For this review, take the finished solid that the model builds, in its own axes (mm). Give positions to 0.01 mm unless a question says otherwise; leave off trailing zeros. Order: outer loops, then holes, each group sorted by start corner. A loop starts at its lowest first (then second) coordinate and runs counter-clockwise, first axis right, second up.
Item 1: The part is to be moulded in two halves that separate along X. For faces 1 (the cylindrical face through (24.369, -22.003, 1.479)), 2 (the cylindrical face through (-29.85, -23.93, 1.52)), 3 (the flat face through (1, -26, 1)), say which applies: released by +X, released by -X, zero draft, split by the parting line, or undercut.
Item 2: For P1, Ø3.5, axis at x = -25, y = -20, coming from the -Z side; P2, Ø5.5, axis at x = -25, y = 20, coming from the -Z side, all flat-tipped, find the tip position at first contact; note any pin that passes through.
Item 3: Consider section D-D (x = 25). Give the boundary of the cut face in (y, z).
Item 4: Consider section B-B (y = 0). Give the boundary of the cut face in (x, z), plus the area to 3 significant figures.
Item 5: Consider section C-C (z = 2). Give the number of separate pieces and of enclosed holes in the cut face, plus the area to 3 significant figures.
Item 6: For probe 1 along Y at (x, z) = (-10, 1); probe 2 along Y at (x, z) = (25, 2.3); probe 3 along X at (y, z) = (0, 1.25), list the stretches that pass through material, from the lowest coordinate up.
Item 7: Consider section A-A (x = 10). Give the boundary of the cut face in (y, z).
Autodesk Inventor part; units mm, degrees
ref_plane "YZ Plane" through (0, 0, 0) normal (1, 0, 0) x (0, 1, 0)
ref_plane "XZ Plane" through (0, 0, 0) normal (0, 1, 0) x (-1, 0, 0)
ref_plane "XY Plane" through (0, 0, 0) normal (0, 0, 1) x (1, 0, 0)
sketch "スケッチ1" plane through (0, 0, 0) normal (0, 0, 1) x (1, 0, 0)
  line L0 (30, -26) -> (-30, -26)
  line L1 (-30, -26) -> (-30, 26)
  line L2 (-30, 26) -> (30, 26)
  line L3 (30, 26) -> (30, -26)
  line L4 (30, -26) -> (-30, 26) construction
  line L5 (-30, -26) -> (30, 26) construction
  point P0 (0, 0)
  dimension "d0" = 60
  dimension "d1" = 52
extrude "押し出し1" add sketch "スケッチ1" along normal blind 3
sketch "スケッチ2" plane through (0, 0, 3) normal (0, 0, 1) x (1, 0, 0)
  line L0 (-10, -20) -> (10, -20)
  line L1 (10, -20) -> (10, 20)
  line L2 (10, 20) -> (-10, 20)
  line L3 (-10, 20) -> (-10, -20)
  line L4 (-10, -20) -> (10, 20) construction
  line L5 (10, -20) -> (-10, 20) construction
  line L6 (-30, -26) -> (30, -26)
  point P0 (0, 0)
  point P1 (0, 20)
  point P2 (0, -20)
  dimension "d4" = 20
  dimension "d5" = 40
  dimension "d6" = 6
hole "穴1" at (-10, 20, 3) at (-10, -20, 3) at (10, -20, 3) at (10, 20, 3) at (0, -20, 3) at (0, 0, 3) at (0, 20, 3) direction (0, 0, -1) diameter 3.3 depth 8.8
sketch "スケッチ4" plane through (0, 0, 3) normal (0, 0, 1) x (1, 0, 0)
  line L0 (-25, -20) -> (25, -20)
  line L1 (25, -20) -> (25, 20)
  line L2 (25, 20) -> (-25, 20)
  line L3 (-25, 20) -> (-25, -20)
  line L4 (-25, -20) -> (25, 20) construction
  line L5 (25, -20) -> (-25, 20) construction
  point P0 (0, 0)
  point P1 (0, 20)
  point P2 (0, -20)
  point P3 (0, 0)
  point P4 (-25, 0)
  point P5 (25, 0)
  dimension "d14" = 50
  dimension "d15" = 40
hole "穴2" at (-25, 20, 3) at (-25, -20, 3) at (25, -20, 3) at (25, 20, 3) at (-25, 0, 3) at (25, 0, 3) direction (0, 0, -1) diameter 4.2 depth 8.8
chamfer "面取り1" distance 2 angle 45 4 edges at (-30, 26, 1.5) (-30, -26, 1.5) (30, -26, 1.5) (30, 26, 1.5)
fillet "フィレット2" radius 2 6 edges at (30, 24, 1.5) (28, 26, 1.5) (-28, 26, 1.5) (-30, 24, 1.5) (-30, -24, 1.5) (-28, -26, 1.5)
sketch "スケッチ5" plane through (0, 0, 3) normal (0, 0, 1) x (1, 0, 0)
  circle A0 centre (-25, 0) radius 2.1
  circle A1 centre (25, -20) radius 2.1
  circle A2 centre (-25, 20) radius 2.1
  circle A3 centre (-25, -20) radius 2.1
  circle A4 centre (25, 20) radius 2.1
  circle A5 centre (25, 0) radius 2.1
  circle A6 centre (0, 0) radius 1.65
  circle A7 centre (10, 20) radius 1.65
  circle A8 centre (-10, -20) radius 1.65
  circle A9 centre (-10, 20) radius 1.65
  circle A10 centre (10, -20) radius 1.65
  circle A11 centre (0, -20) radius 1.65
  circle A12 centre (0, 20) radius 1.65
  arc A13 (-28.5858, -25.4142) -> (-27.1716, -26) centre (-27.1716, -24) ccw
  line L0 (-27.1716, -26) -> (28, -26)
  line L1 (30, -24) -> (28, -26)
  line L2 (30, -24) -> (30, 23.1716)
  arc A14 (30, 23.1716) -> (29.4142, 24.5858) centre (28, 23.1716) ccw
  line L3 (28.5858, 25.4142) -> (29.4142, 24.5858)
  arc A15 (28.5858, 25.4142) -> (27.1716, 26) centre (27.1716, 24) ccw
  line L4 (27.1716, 26) -> (-27.1716, 26)
  arc A16 (-27.1716, 26) -> (-28.5858, 25.4142) centre (-27.1716, 24) ccw
  line L5 (-29.4142, 24.5858) -> (-28.5858, 25.4142)
  arc A17 (-29.4142, 24.5858) -> (-30, 23.1716) centre (-28, 23.1716) ccw
  line L6 (-30, 23.1716) -> (-30, -23.1716)
  arc A18 (-30, -23.1716) -> (-29.4142, -24.5858) centre (-28, -23.1716) ccw
  line L7 (-28.5858, -25.4142) -> (-29.4142, -24.5858)
  point P0 (0, 0)
properties part number "Diode_laser_Mount"
Resolved:
1. face 1: undercut
1. face 2: released by -X
1. face 3: zero draft
2. P1: passes through
2. P2: stops at z = 0
3. outline: (-26, 0) - (-22.1, 0) - (-22.1, 3) - (-26, 3) - close; (-17.9, 0) - (-2.1, 0) - (-2.1, 3) - (-17.9, 3) - close; (2.1, 0) - (17.9, 0) - (17.9, 3) - (2.1, 3) - close; (22.1, 0) - (26, 0) - (26, 3) - (22.1, 3) - close
4. outline: (-30, 0) - (-27.1, 0) - (-27.1, 3) - (-30, 3) - close; (-22.9, 0) - (-1.65, 0) - (-1.65, 3) - (-22.9, 3) - close; (1.65, 0) - (22.9, 0) - (22.9, 3) - (1.65, 3) - close; (27.1, 0) - (30, 0) - (30, 3) - (27.1, 3) - close
4. area: 145 mm2
5. separate pieces: 1
5. enclosed holes: 13
5. area: 2,970 mm2
6. probe 1: y = -26 to -21.65, -18.35 to 18.35, 21.65 to 26
6. probe 2: y = -26 to -22.1, -17.9 to -2.1, 2.1 to 17.9, 22.1 to 26
6. probe 3: x = -30 to -27.1, -22.9 to -1.65, 1.65 to 22.9, 27.1 to 30
7. outline: (-26, 0) - (-21.65, 0) - (-21.65, 3) - (-26, 3) - close; (-18.35, 0) - (18.35, 0) - (18.35, 3) - (-18.35, 3) - close; (21.65, 0) - (26, 0) - (26, 3) - (21.65, 3) - close
